from build123d import *

# Parameters (mm, degrees)
SKETCH1_R                               = 8
BOSS_EXTRUDE1_DEPTH                     = 10
SKETCH3_R                               = 3.5
CUT_EXTRUDE2_DEPTH                      = 179.204938203
SKETCH4_R                               = 6
CUT_EXTRUDE3_DEPTH                      = 6
CIRPATTERN4_COUNT                       = 6
TAP_DRILL_FOR_M10X1_25_TAP1_D           = 8.8
TAP_DRILL_FOR_M10X1_25_TAP1_DEPTH       = 24
TAP_DRILL_FOR_M10X1_25_TAP1_CSINK_D     = 8.85
TAP_DRILL_FOR_M10X1_25_TAP1_CSINK_ANGLE = 90
TAP_DRILL_FOR_M10X1_25_TAP1_TIP         = 2.643786724
SKETCH10_R                              = 12.5
CUT_EXTRUDE4_DEPTH                      = 10


with BuildPart() as part:
    # Sketch1 → Boss-Extrude1 (new, symmetric)
    with BuildSketch(Plane.XY):
        with BuildLine():
            Line((46, 125), (46, 0))
            Line((46, 0), (-46, 0))
            Line((-46, 0), (-46, 125))
            ThreePointArc((-46, 125), (0, 171), (46, 125))
        make_face()
        with Locations((0, 125)):
            Circle(SKETCH1_R, mode=Mode.SUBTRACT)
    extrude(amount=BOSS_EXTRUDE1_DEPTH, both=True)

    # Sketch3 → Cut-Extrude2 (cut, through all)
    with BuildSketch(Plane.XY.offset(10)):
        with Locations((0, 161)):
            Circle(SKETCH3_R)
    cut_extrude2 = extrude(amount=-CUT_EXTRUDE2_DEPTH, mode=Mode.SUBTRACT)

    # Sketch4 → Cut-Extrude3 (cut)
    with BuildSketch(Plane.XY.offset(10)):
        with Locations((0, 161)):
            Circle(SKETCH4_R)
    cut_extrude3 = extrude(amount=-CUT_EXTRUDE3_DEPTH, mode=Mode.SUBTRACT)

    # CirPattern4: Cut-Extrude2, Cut-Extrude3 ×6 about axis
    cirpattern4_axis = Axis((0, 125, 0), (0, 0, 1))
    add([cut_extrude2.rotate(cirpattern4_axis, i * 360 / CIRPATTERN4_COUNT) for i in range(1, CIRPATTERN4_COUNT)], mode=Mode.SUBTRACT)
    add([cut_extrude3.rotate(cirpattern4_axis, i * 360 / CIRPATTERN4_COUNT) for i in range(1, CIRPATTERN4_COUNT)], mode=Mode.SUBTRACT)

    # Tap Drill for M10x1.25 Tap1
    with Locations(Plane(origin=(0, 0, 0), x_dir=(-1, 0, 0), z_dir=(0, -1, 0))):
        with Locations((-30, 0), (30, 0)):
            CounterSinkHole(TAP_DRILL_FOR_M10X1_25_TAP1_D / 2, TAP_DRILL_FOR_M10X1_25_TAP1_CSINK_D / 2, depth=TAP_DRILL_FOR_M10X1_25_TAP1_DEPTH, counter_sink_angle=TAP_DRILL_FOR_M10X1_25_TAP1_CSINK_ANGLE)
            with Locations((0, 0, -(TAP_DRILL_FOR_M10X1_25_TAP1_DEPTH + TAP_DRILL_FOR_M10X1_25_TAP1_TIP / 2))):  # 118° drill point
                Cone(0, TAP_DRILL_FOR_M10X1_25_TAP1_D / 2, TAP_DRILL_FOR_M10X1_25_TAP1_TIP, mode=Mode.SUBTRACT)

    # Sketch10 → Cut-Extrude4 (cut)
    with BuildSketch(Plane(origin=(0, 0, -10), x_dir=(-1, 0, 0), z_dir=(0, 0, -1))):
        with Locations((0, 125)):
            Circle(SKETCH10_R)
    extrude(amount=-CUT_EXTRUDE4_DEPTH, mode=Mode.SUBTRACT)


solid = part.part
Here's how the part is built. I have some questions about the finished solid (model axes, mm). A direction names the side the tool comes from. Coordinates: 2 decimals unless noted, no trailing zeros. Write each loop counter-clockwise with the first axis right and the second up, starting at its lowest first coordinate (ties: lowest second). Pieces come first, ordered by that corner, then holes.
1) Thinking about a two-plate mould opening in X: for faces 1 (the face through (31.96, 137.05, 7.04)), 2 (the face through (46, 63, 0)), 3 (the face through (-25.936, 12.18, 1.685)), 4 (the face through (1, 0, 0)), which applies, +X half, -X half, draft (parallel to the pull), parting line (faces both ways), or undercut?
Filled in:
face 1: undercut
face 2: +X half
face 3: undercut
face 4: draft
2) If we section it at C-C (y = 161): List the corners of the cut face in (x, z) for me, plus the area to 3 significant figures.
Filled in:
outline: (-28.64, -10) - (-3.5, -10) - (-3.5, 4) - (-6, 4) - (-6, 10) - (-28.64, 10) - close; (3.5, -10) - (28.64, -10) - (28.64, 10) - (6, 10) - (6, 4) - (3.5, 4) - close
area: 975 mm2
3) If I drill on line 1 (Y direction, x = -33.5, z = 4.25); line 2 (Z direction, x = 30, y = 13.25); line 3 (Y direction, x = 0, z = -5.5), over which ranges is the centre line in solid material (lowest first)?
Filled in:
line 1: y = 0 to 101.47, 112.53 to 137.47, 148.53 to 156.52
line 2: z = -10 to -4.4, 4.4 to 10
line 3: y = 0 to 85.5, 92.5 to 112.5, 137.5 to 157.5, 164.5 to 171
4) If we section it at A-A (y = 107): List the corners of the cut face in (x, z) for me, plus the area to 3 significant figures.
Filled in:
outline: (-46, -10) - (-34.68, -10) - (-34.68, 4) - (-37.18, 4) - (-37.18, 10) - (-46, 10) - close; (-27.68, -10) - (27.68, -10) - (27.68, 4) - (25.18, 4) - (25.18, 10) - (-25.18, 10) - (-25.18, 4) - (-27.68, 4) - close; (34.68, -10) - (46, -10) - (46, 10) - (37.18, 10) - (37.18, 4) - (34.68, 4) - close
area: 1,500 mm2
5) Which directions (+Z, -Z, +X, -X, +Y, -Y) give clear straight access to the entire face, cutting with the end or side of a thin tool? Please do faces 5 (the face through (-31.96, 112.95, 7.04)), 6 (the face through (-46, 62, 0)).
Filled in:
face 5: +Z
face 6: +Z, -Z, -X, +Y, -Y
6) If we section it at D-D (y = 11): List the corners of the cut face in (x, z) for me.
Filled in:
outline: (-46, -10) - (46, -10) - (46, 10) - (-46, 10) - close; hole circle Ø8.8 at (-30, 0); hole circle Ø8.8 at (30, 0)
7) I'm going to push flat-ended pins straight in: pin 1 (6 mm diameter, centred on x = 10, z = 4.5, fed in from +Y); pin 2 (9 mm diameter, centred on x = 31.18, y = 143, fed in from +Z); pin 3 (1.5 mm diameter, centred on x = -15.5, z = -2, fed in from +Y). Where does each tip first touch, or does it pass through?
Filled in:
pin 1: stops at y = 170.46
pin 2: stops at z = 4
pin 3: stops at y = 168.57
8) If we section it at B-B (z = -8.25): List the corners of the cut face in (x, y) for me.
Filled in:
outline: (-46, 0) - (46, 0) - (46, 125) arc R46 ccw to (-46, 125) - close; hole circle Ø7 at (-31.18, 107); hole circle Ø7 at (-31.18, 143); hole circle Ø25 at (0, 125); hole circle Ø7 at (0, 89); hole circle Ø7 at (0, 161); hole circle Ø7 at (31.18, 107); hole circle Ø7 at (31.18, 143)
